from build123d import *

# Parameters (mm, degrees)
F1_DEPTH = 26
F2_W     = 3
F2_H     = 301.5
F3_DEPTH = 10


with BuildPart() as f1:
    # F0 (on Top) → F1 (new body)
    with BuildSketch(Plane.XY):
        Polygon((603, 0), (0, 0), (0, -904.5), (904.5, -904.5), (904.5, -601.5), (603, -601.5), align=None)
    extrude(amount=F1_DEPTH)

    # F2 (on face) → F3 (cut)
    with BuildSketch(Plane.XY.offset(26)):
        Polygon((0, -600), (0, -603), (301.5, -603), (304.5, -603), (904.5, -603), (904.5, -600), align=None)
        with Locations((303, -753.75)):
            Rectangle(F2_W, F2_H)
    extrude(amount=-F3_DEPTH, mode=Mode.SUBTRACT)


solid = f1.part
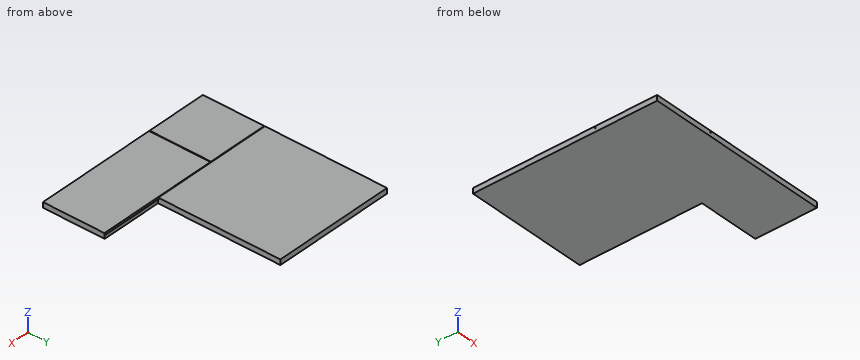
For this review, take the finished solid that the model builds, in its own axes (mm). Coordinates: 2 decimals unless noted, no trailing zeros. Loops run counter-clockwise (first coordinate to the right, second up) from the corner with the lowest first, then second, coordinate; pieces in that order, holes last. Notation, with made-up numbers: (-21, 27.25) -> (-3, 27.25) arc R11 ccw to (-3, 42.25) -> close; hole circle Ø7 at (75.25, -4.75). An arc over 180 degrees is marked (long way). Write each question's results on one line, items separated by ' | '.
Q1. Add section B-B, the plane y = -112.5. State the section outline as (x, z) points.
Taken from the geometry:
outline: (0, 0) -> (603, 0) -> (603, 26) -> (0, 26) -> close
Q2. For pin 1 Ø4 at (y, z) = (-201.5, 7) entering from +X; pin 2 Ø5 at (x, z) = (721, 23) entering from +Y; pin 3 Ø4 at (x, z) = (775, 6.5) entering from +Y, all flat-tipped, find the tip position at first contact; note any pin that passes through.
Taken from the geometry:
pin 1: x = 603 | pin 2: y = -603 | pin 3: y = -601.5
Q3. Add section A-A, the plane z = 21.5. State the section outline as (x, y) points.
Taken from the geometry:
outline: (0, -904.5) -> (301.5, -904.5) -> (301.5, -603) -> (0, -603) -> close; (0, -600) -> (603, -600) -> (603, 0) -> (0, 0) -> close; (304.5, -904.5) -> (904.5, -904.5) -> (904.5, -603) -> (304.5, -603) -> close
Q4. To check wall thickness, follow line 1 along Y through (x, z) = (474.5, 19); line 2 along Y through (x, z) = (860, 2.5); line 3 along X through (y, z) = (-618, 17.5). State the ranges of each line that lie inside material, in increasing order. Write a range as [from, to].
Taken from the geometry:
line 1: [-904.5, -603], [-600, 0] | line 2: [-904.5, -601.5] | line 3: [0, 301.5], [304.5, 904.5]
